Autodesk Fusion 360 part; units mm, degrees
sketch "Sketch1" plane through (0, 0, 0) normal (1, 0, 0) x (0, 1, 0)
  line L0 (0, 0) -> (55, 0)
  line L1 (55, 0) -> (55, 20)
  line L2 (55, 20) -> (0, 20)
  line L3 (0, 20) -> (0, 0)
sketch "Sketch2" plane through (0, 0, 0) normal (1, 0, 0) x (0, 1, 0)
  circle A0 centre (27.5766, 10.2067) radius 6.35
  dimension "d1" = 12.7
extrude "Extrude1" add sketch "Sketch1" along normal blind 2
hole "Hole1" at (2, 27.5, 10) direction (-1, 0, 0) diameter 12.7 depth 8 tip angle 118
sketch "Sketch3" plane through (2, 0, 0) normal (1, 0, 0) x (0, 1, 0)
  circle A0 centre (27.5, 10) radius 6.35
  line L0 (0, 20) -> (0, 0)
  line L1 (0, 0) -> (55, 0)
  line L2 (55, 0) -> (55, 20)
  line L3 (55, 20) -> (0, 20)
  circle A1 centre (27.5, 10) radius 8.2006
  circle A2 centre (27.5, 10) radius 6.35
extrude "Extrude2" add sketch "Sketch3" along normal blind 21 contours A1
hole "Hole2" at (2, 9.5562, 8.4294) direction (-1, 0, 0) diameter 6.5 depth 8 tip angle 118
hole "Hole3" at (2, 44.397, 7.8265) direction (-1, 0, 0) diameter 6.5 depth 8 tip angle 118
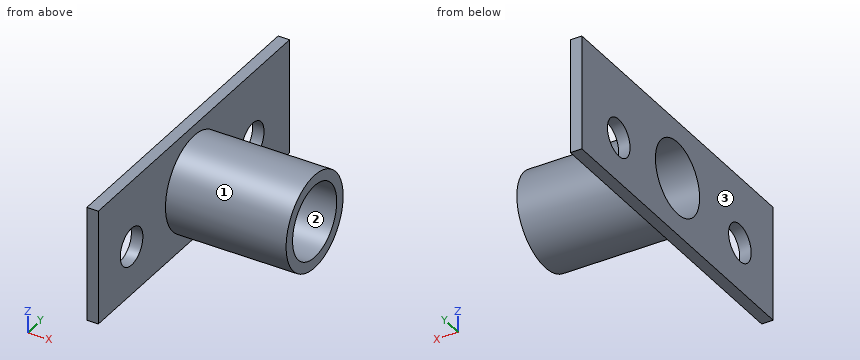
Read the model definition and answer for the solid it produces. Units are mm, in the model's axes. Face numbers are marked on the shaded views. Coordinates: 2 decimals unless noted, no trailing zeros. Write each loop counter-clockwise with the first axis right and the second up, starting at its lowest first coordinate (ties: lowest second). Pieces come first, ordered by that corner, then holes. Notation, with made-up numbers: (35.25, -10.75) -> (67.25, -10.75) arc R35 ccw to (67.25, 24.25) -> close; hole circle Ø9 at (-29, 35.25). An arc over 180 degrees is marked (long way). Write item = value, one per line.
(1) Straight lines are drawn through the part: L1, parallel to Z at x = 16, y = 27.5; L2, parallel to X at y = 20, z = 5.25; L3, parallel to Y at x = 10.25, z = 13.25. For each, find the intervals that lie inside material, in ascending order. Write a range as from..to.
From the geometry:
L1 = 1.8..3.65, 16.35..18.2
L2 = 0..2
L3 = 19.97..22.04, 32.96..35.03
(2) Section A-A on y = 27.5 is taken. Write down the section's boundary in (x, z), plus the area to 3 significant figures.
From the geometry:
outline = (0, 0) -> (2, 0) -> (2, 1.8) -> (23, 1.8) -> (23, 3.65) -> (0, 3.65) -> close; (0, 16.35) -> (23, 16.35) -> (23, 18.2) -> (2, 18.2) -> (2, 20) -> (0, 20) -> close
area = 92.3 mm2
(3) For a pull along Y with two mould halves and no side action, classify the marked faces 1, 2 and 3 as +Y half, -Y half, draft (parallel to the pull), parting line (faces both ways), or undercut.
From the geometry:
face_1 = parting line
face_2 = undercut
face_3 = draft
(4) Given pin 1 Ø1.5 at (y, z) = (10.5, 15) entering from +X; pin 2 Ø5 at (x, z) = (15, 3.5) entering from -Y; pin 3 Ø1 at (x, z) = (18.5, 10.5) entering from -Y, each flat-ended and moving along its own axis, determine where each tip first touches the part or whether it passes through.
From the geometry:
pin_1 = 2
pin_2 = 20.34
pin_3 = 19.3
(5) Section D-D on x = 15.5 is taken. Write down the section's boundary in (y, z), plus the area to 3 significant figures.
From the geometry:
outline = circle Ø16.4 at (27.5, 10); hole circle Ø12.7 at (27.5, 10)
area = 84.6 mm2
(6) Section B-B on z = 8 is taken. Write down the section's boundary in (x, y), plus the area to 3 significant figures.
From the geometry:
outline = (0, 0) -> (2, 0) -> (2, 6.33) -> (0, 6.33) -> close; (0, 12.78) -> (2, 12.78) -> (2, 19.55) -> (23, 19.55) -> (23, 21.47) -> (0, 21.47) -> close; (0, 33.53) -> (23, 33.53) -> (23, 35.45) -> (2, 35.45) -> (2, 41.15) -> (0, 41.15) -> close; (0, 47.64) -> (2, 47.64) -> (2, 55) -> (0, 55) -> close
area = 141 mm2
(7) Section C-C on z = 14.5 is taken. Write down the section's boundary in (x, y).
From the geometry:
outline = (0, 0) -> (2, 0) -> (2, 20.64) -> (23, 20.64) -> (23, 23.02) -> (0, 23.02) -> close; (0, 31.98) -> (23, 31.98) -> (23, 34.36) -> (2, 34.36) -> (2, 55) -> (0, 55) -> close
